from build123d import *

# Parameters (mm, degrees)
SKETCH9_R          = 8.1
BASE_FLANGE2_DEPTH = 4


# Sheet-metal steps are written as plain solids
with BuildPart() as part:
    # Sketch9 → Base-Flange2 (new body)
    with BuildSketch(Plane.XY):
        with BuildLine():
            Line((-155, -235), (155, -235))
            Line((155, -235), (155, -54.5))
            ThreePointArc((155, -54.5), (156.171572875, -51.671572875), (159, -50.5))
            Line((159, -50.5), (242, -50.5))
            ThreePointArc((242, -50.5), (244.828427125, -49.328427125), (246, -46.5))
            Line((246, -46.5), (246, 46.5))
            ThreePointArc((246, 46.5), (244.828427125, 49.328427125), (242, 50.5))
            Line((242, 50.5), (159, 50.5))
            ThreePointArc((159, 50.5), (156.171572875, 51.671572875), (155, 54.5))
            Line((155, 54.5), (155, 235))
            Line((155, 235), (-155, 235))
            Line((-155, 235), (-155, -235))
        make_face()
        with Locations((-95, 150.5)):
            Circle(SKETCH9_R, mode=Mode.SUBTRACT)
        with Locations((-95, -150.5)):
            Circle(SKETCH9_R, mode=Mode.SUBTRACT)
        with BuildLine():
            Line((159, 40.5), (232, 40.5))
            ThreePointArc((232, 40.5), (234.828427125, 39.328427125), (236, 36.5))
            Line((236, 36.5), (236, -36.5))
            ThreePointArc((236, -36.5), (234.828427125, -39.328427125), (232, -40.5))
            Line((232, -40.5), (159, -40.5))
            ThreePointArc((159, -40.5), (156.171572875, -39.328427125), (155, -36.5))
            Line((155, -36.5), (155, 36.5))
            ThreePointArc((155, 36.5), (156.171572875, 39.328427125), (159, 40.5))
        make_face(mode=Mode.SUBTRACT)
    extrude(amount=-BASE_FLANGE2_DEPTH)


solid = part.part
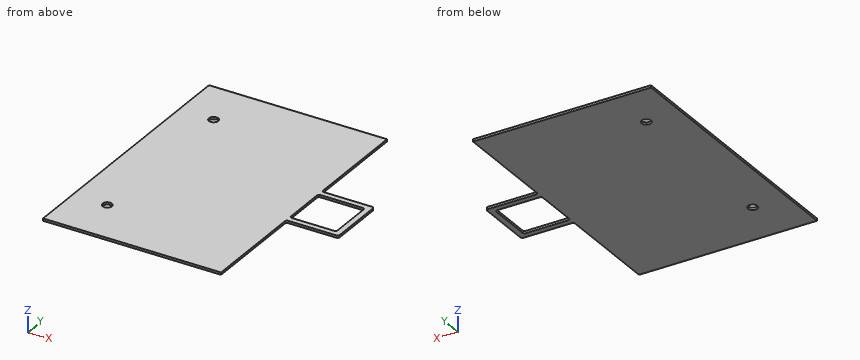
Can you work these out from the model? Positions are in its coordinate system, mm. Give positions to 0.01 mm unless a question says otherwise; leave off trailing zeros. Order: outer loops, then holes, each group sorted by start corner. A loop starts at its lowest first (then second) coordinate and runs counter-clockwise, first axis right, second up. Notation, with made-up numbers: M -24,-33 L -10,-33 A7 ccw -10,-28 Z; hole C 67.25,27.25 d3. An arc over 180 degrees is marked long. Use one line per item in the form item = value.
Item 1: If we section it at A-A, the plane x = -95: Write out the boundary of the cut face in (y, z), and give its area (3 significant figures).
Values follow:
outline = M -235,-4 L -158.6,-4 L -158.6,0 L -235,0 Z; M -142.4,-4 L 142.4,-4 L 142.4,0 L -142.4,0 Z; M 158.6,-4 L 235,-4 L 235,0 L 158.6,0 Z
area = 1,750 mm^2
Item 2: If we section it at D-D, the plane y = -23.5: Write out the boundary of the cut face in (x, z).
Values follow:
outline = M -155,-4 L 155,-4 L 155,0 L -155,0 Z; M 236,-4 L 246,-4 L 246,0 L 236,0 Z
Item 3: Will these pins go through, and if not, where does the flat tip stop? pin 1 Ø14.5 at (x, y) = (-95, -150.5) entering from +Z; pin 2 Ø1 at (y, z) = (-90, -2.5) entering from +X; pin 3 Ø2 at (x, z) = (195.5, -2.5) entering from +Y; pin 4 Ø2 at (x, z) = (182, -2) entering from -Y.
Values follow:
pin_1 = through
pin_2 = 155
pin_3 = 50.5
pin_4 = -50.5
Item 4: If I drill on line 1 along Y through (x, z) = (-95, -2.55); line 2 along Y through (x, z) = (-99, -1.6); line 3 along X through (y, z) = (-36, -1), over which ranges is the centre line in solid material (lowest first)? Write a range as [from, to].
Values follow:
line_1 = [-235, -158.6], [-142.4, 142.4], [158.6, 235]
line_2 = [-235, -157.54], [-143.46, 143.46], [157.54, 235]
line_3 = [-155, 155], [236, 246]
Item 5: If we section it at C-C, the plane y = -150.5: Write out the boundary of the cut face in (x, z), and give its area (3 significant figures).
Values follow:
outline = M -155,-4 L -103.1,-4 L -103.1,0 L -155,0 Z; M -86.9,-4 L 155,-4 L 155,0 L -86.9,0 Z
area = 1,180 mm^2
Item 6: If we section it at B-B, the plane z = -3: Write out the boundary of the cut face in (x, y), and give its area (3 significant figures).
Values follow:
outline = M -155,-235 L 155,-235 L 155,-54.5 A4 cw 159,-50.5 L 242,-50.5 A4 ccw 246,-46.5 L 246,46.5 A4 ccw 242,50.5 L 159,50.5 A4 cw 155,54.5 L 155,235 L -155,235 Z; hole C -95,-150.5 d16.2; hole C -95,150.5 d16.2; hole M 155,-36.5 A4 ccw 159,-40.5 L 232,-40.5 A4 ccw 236,-36.5 L 236,36.5 A4 ccw 232,40.5 L 159,40.5 A4 ccw 155,36.5 Z
area = 148,000 mm^2
